```python
from build123d import *

# Parameters (mm, degrees)
BOSS_EXTRUDE1_DEPTH = 15
BOSS_EXTRUDE2_DEPTH = 40
BOSS_EXTRUDE3_DEPTH = 15
SKETCH5_R           = 4.95
CUT_EXTRUDE1_DEPTH  = 15
CUT_EXTRUDE2_START  = -15
SKETCH6_R           = 4.95
CUT_EXTRUDE2_DEPTH  = 15
SKETCH7_W           = 1.5
SKETCH7_H           = 10
CUT_EXTRUDE3_DEPTH  = 76
SKETCH8_W           = 50
SKETCH8_H           = 2.5
CUT_EXTRUDE4_DEPTH  = 76


with BuildPart() as part:
    # Sketch2 → Boss-Extrude1 (new body)
    with BuildSketch(Plane.XY):
        with BuildLine():
            Line((-5, 10), (-15, 10))
            ThreePointArc((-15, 10), (-22.071067812, -7.071067812), (-5, 0))
            Line((-5, 0), (5, 0))
            ThreePointArc((5, 0), (22.071067812, -7.071067812), (15, 10))
            Line((15, 10), (5, 10))
            Line((5, 10), (-5, 10))
        make_face()
    extrude(amount=BOSS_EXTRUDE1_DEPTH)

    # Sketch3 → Boss-Extrude2 (add)
    with BuildSketch(Plane.XY.offset(15)):
        Polygon((-11.5, 0), (-15, 10), (15, 10), (11.5, 0), align=None)
    extrude(amount=BOSS_EXTRUDE2_DEPTH)

    # Sketch4 → Boss-Extrude3 (add)
    with BuildSketch(Plane.XY.offset(55)):
        with BuildLine():
            Line((-5, 10), (-15, 10))
            ThreePointArc((-15, 10), (-22.071067812, -7.071067812), (-5, 0))
            Line((-5, 0), (5, 0))
            ThreePointArc((5, 0), (22.071067812, -7.071067812), (15, 10))
            Line((15, 10), (5, 10))
            Line((5, 10), (-5, 10))
        make_face()
    extrude(amount=BOSS_EXTRUDE3_DEPTH)

    # Sketch5 → Cut-Extrude1 (cut)
    with BuildSketch(Plane(origin=(0, 0, 0), x_dir=(-1, 0, 0), z_dir=(0, 0, -1))):
        with Locations((15, 0)):
            Circle(SKETCH5_R)
        with Locations((-15, 0)):
            Circle(SKETCH5_R)
    extrude(amount=-CUT_EXTRUDE1_DEPTH, mode=Mode.SUBTRACT)

    # Sketch6 → Cut-Extrude2 (cut)
    with BuildSketch(Plane.XY.offset(70).offset(CUT_EXTRUDE2_START)):
        with Locations(Location((-15, 0, 0), (0, 0, 180))):
            Circle(SKETCH6_R)
        with Locations(Location((15, 0, 0), (0, 0, 180))):
            Circle(SKETCH6_R)
    extrude(amount=CUT_EXTRUDE2_DEPTH, mode=Mode.SUBTRACT)

    # Sketch7 → Cut-Extrude3 (cut, through all)
    with BuildSketch(Plane.XY.offset(70)):
        with Locations((-15, -5)):
            Rectangle(SKETCH7_W, SKETCH7_H)
        with Locations((15, -5)):
            Rectangle(SKETCH7_W, SKETCH7_H)
    extrude(amount=-CUT_EXTRUDE3_DEPTH, mode=Mode.SUBTRACT)

    # Sketch8 → Cut-Extrude4 (cut, through all)
    with BuildSketch(Plane(origin=(0, 0, 0), x_dir=(-1, 0, 0), z_dir=(0, 0, -1))):
        with Locations((0, 8.75)):
            Rectangle(SKETCH8_W, SKETCH8_H)
    extrude(amount=-CUT_EXTRUDE4_DEPTH, mode=Mode.SUBTRACT)


solid = part.part
```
CAD build for the part. Positions are in the model's coordinates, mm. A direction names the side the tool comes from. Round coordinates to 2 decimals unless told otherwise and drop trailing zeros. Order: outer loops, then holes, each group sorted by start corner. A loop starts at its lowest first (then second) coordinate and runs counter-clockwise, first axis right, second up. Notation, with made-up numbers: (29.5, 0.25) - (34.5, 0.25) arc R20 ccw to (34.5, 28.25) - close; hole circle Ø8 at (54.5, -37). An arc over 180 degrees is marked (long way). Answer as CSV lines item,"result". Start each with the question number.
1. Saw through at D-D, the plane z = 49. Write the cut outline in (x, y) (3 decimals).
2. Saw through at B-B, the plane z = 62.5. Write the cut outline in (x, y).
3. Saw through at A-A, the plane x = 15. Write the cut outline in (y, z), and give its area (3 significant figures).
4. Drill centre lines: L1, parallel to Z at x = -6, y = -3.75; L2, parallel to Y at x = 15, z = 6; L3, parallel to Y at x = 4.5, z = 61. Where is each one in solid material? Low to high. Write a range as [from, to].
5. Saw through at C-C, the plane y = -1.25. Count the separate pieces of the cut face and the enclosed holes in it, and give its area (3 significant figures).
6. Tool access for faces 4 (the face through (-7.74, -6.877, 62.395)), 5 (the face through (-12.794, 3.698, 34.72)), 6 (the face through (10, -5, 15)), 7 (the face through (-12, 2, 15)): list every direction of +Z, -Z, +X, -X, +Y, -Y with a clear straight run to the whole face (end or side of a thin tool).
7. Pull direction Y, two halves, no side cores. Call faces 1 (the face through (-12, 2, 55)), 2 (the face through (0, 0, 35)), 3 (the face through (-20.5, -1.1, 15)): +Y half, -Y half, draft (parallel to the pull), parting line (faces both ways), or undercut.
8. Pin check, flat tips, straight feed: pin 1 (1.5 mm diameter, centred on y = -4.5, z = 11.5, fed in from +X); pin 2 (8 mm diameter, centred on y = -3.5, z = 56.5, fed in from +X); pin 3 (0.9 mm diameter, centred on x = -11.5, y = 1.5, fed in from +Z); pin 4 (5.5 mm diameter, centred on y = -7, z = 63.5, fed in from +X). Stop position of each tip, or through.
Model answer:
1,outline,"(-14.125, 7.5) - (-11.5, 0) - (11.5, 0) - (14.125, 7.5) - close"
2,outline,"(-21.61, 7.5) arc R10 ccw to (-15.75, -9.97) - (-15.75, -4.89) arc R4.95 cw (long way) to (-14.25, -4.89) - (-14.25, -9.97) arc R10 ccw to (-5, 0) - (5, 0) arc R10 ccw to (14.25, -9.97) - (14.25, -4.89) arc R4.95 cw (long way) to (15.75, -4.89) - (15.75, -9.97) arc R10 ccw to (21.61, 7.5) - close"
3,outline,"(4.95, 0) - (7.5, 0) - (7.5, 15) - (4.95, 15) - close; (4.95, 55) - (7.5, 55) - (7.5, 70) - (4.95, 70) - close"
3,area,"76.5 mm²"
4,L1,"z = [0, 15], [55, 70]"
4,L2,"y = [4.95, 7.5]"
4,L3,"y = [0, 7.5]"
5,separate pieces,"8"
5,enclosed holes,"0"
5,area,"616 mm²"
6,face 4,"+Z, -Z, -Y"
6,face 5,"-X, -Y"
6,face 6,"+X, -X, -Y"
6,face 7,"-Z"
7,face 1,"undercut"
7,face 2,"-Y half"
7,face 3,"draft"
8,pin 1,"stops at x = 24.27"
8,pin 2,"stops at x = 25"
8,pin 3,"stops at z = 55"
8,pin 4,"stops at x = 24.05"
